Job drawing, mm, ordinate dimensions from the low corner. One solid piece. A direction names the side the tool comes from. Coordinates: 2 decimals unless noted, no trailing zeros. Write each loop counter-clockwise with the first axis right and the second up, starting at its lowest first coordinate (ties: lowest second). Pieces come first, ordered by that corner, then holes. Notation, with made-up numbers: M 9.5,8.25 L 18.5,8.25 A27 cw 18.5,38.25 Z; hole C -26.5,-3 d11. An arc over 180 degrees is marked long. Answer as CSV lines item,"result". Start each with the question number.
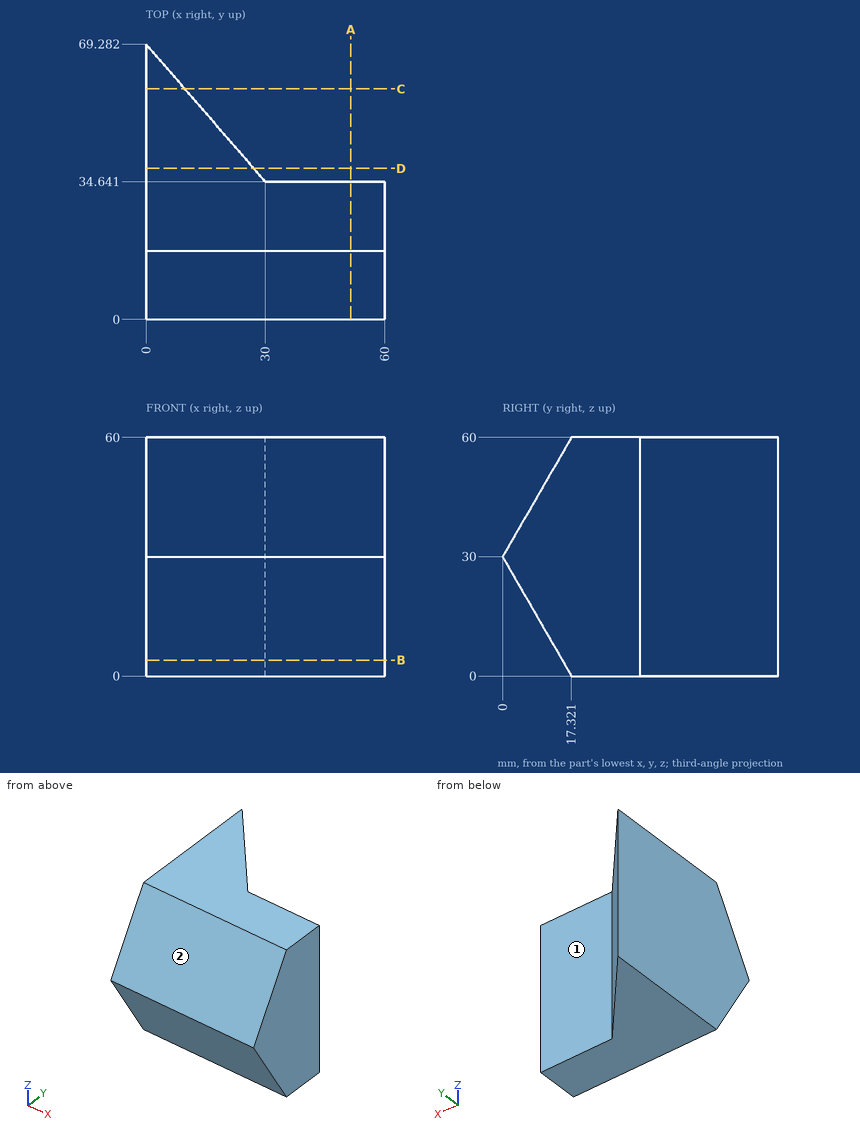
1) Band-saw the part on C-C, the plane y = 58. List the corners of the cut face in (x, z), plus the area to 3 significant figures.
2) Band-saw the part on D-D, the plane y = 38. List the corners of the cut face in (x, z), plus the area to 3 significant figures.
3) Probe L1, parallel to Z at x = 34.5, y = 5.5 (1 decimal); L2, parallel to Y at x = 47, z = 16 (1 decimal); L3, parallel to Y at x = 15, z = 15. List the from-to ranges inside material, lowest first. Write a range as [from, to].
4) Pin check, flat tips, straight feed: P1, Ø12, axis at x = 16, z = 18.5, coming from the -Y side (1 decimal); P2, Ø9, axis at x = 46.5, z = 27.5, coming from the +Y side; P3, Ø8, axis at x = 22.5, z = 52.5, coming from the +Y side. Stop position of each tip, or through.
5) Tool access for the marked faces 1 and 2: list every direction of +Z, -Z, +X, -X, +Y, -Y with a clear straight run to the whole face (end or side of a thin tool).
6) Band-saw the part on B-B, the plane z = 4. List the corners of the cut face in (x, y), plus the area to 3 significant figures.
7) Band-saw the part on A-A, the plane x = 51.5. List the corners of the cut face in (y, z), plus the area to 3 significant figures.
Result sheet:
1,outline,"M 0,0 L 9.77,0 L 9.77,60 L 0,60 Z"
1,area,"586 mm²"
2,outline,"M 0,0 L 27.09,0 L 27.09,60 L 0,60 Z"
2,area,"1,630 mm²"
3,L1,"z = [20.5, 39.5]"
3,L2,"y = [8.1, 34.6]"
3,L3,"y = [8.66, 51.96]"
4,P1,"stops at y = 3.2"
4,P2,"stops at y = 34.64"
4,P3,"stops at y = 47.92"
5,face 1,"+Z, -Z, +X, +Y"
5,face 2,"+Z, +X, -X, -Y"
6,outline,"M 0,15.01 L 60,15.01 L 60,34.64 L 30,34.64 L 0,69.28 Z"
6,area,"1,700 mm²"
7,outline,"M 0,30 L 17.32,0 L 34.64,0 L 34.64,60 L 17.32,60 Z"
7,area,"1,560 mm²"
